Here's how the part is built. I have some questions about the finished solid (model axes, mm). Face numbers are marked on the shaded views. A direction names the side the tool comes from. Give positions to 0.01 mm unless a question says otherwise; leave off trailing zeros. Loops run counter-clockwise (first coordinate to the right, second up) from the corner with the lowest first, then second, coordinate; pieces in that order, holes last. Notation, with made-up numbers: (48.5, -30) - (106.5, -30) arc R19 ccw to (106.5, -2) - close; hole circle Ø6 at (30.5, 26.5). An arc over 180 degrees is marked (long way). Return JSON: item names as keys, results as strings. Group by question number.
(1) For P1, Ø2.5, axis at x = 6.35, z = 0, coming from the -Y side (3 decimals); P2, Ø1.5, axis at x = 11.5, y = 2.5, coming from the +Z side; P3, Ø5, axis at x = 27, y = 3, coming from the -Z side, each with a flat end and sliding along its axis, tell me the tip position at first contact or that it passes through.
(2) If we section it at C-C (x = 6.35): Please give me the cut outline in (y, z) (3 decimals).
(3) I need wall thicknesses on probe 1 along X at (y, z) = (2.85, 0); probe 2 along X at (y, z) = (-1.4, 0); probe 3 along X at (y, z) = (2.25, 0.5). Which ranges of each line are inside material? Lowest first, please. Write a range as [from, to].
(4) If we section it at B-B (y = 3.5): Please give me the cut outline in (x, z) (3 decimals).
(5) If we section it at A-A (z = 0): Please give me the cut outline in (x, y) (1 decimal), then the cut area to 3 significant figures.
(6) If we section it at D-D (x = 32.5): Please give me the cut outline in (y, z) (1 decimal).
(7) On a 3-axis mill with a long thin cutter (end or side, diameter ignored), from which of +Z, -Z, +X, -X, +Y, -Y can I reach the whole of each face in a straight line? I mean the marked faces 1 and 2. Say none if no direction works.
```python
from build123d import *

# Parameters (mm, degrees)
SKETCH1_R               = 4.7625
BOSS_EXTRUDE1_DEPTH     = 38.1
SKETCH2_R               = 2.0066
CUT_EXTRUDE1_DEPTH      = 7.9248
SKETCH3_R               = 1.1303
CUT_EXTRUDE2_DEPTH      = 8.6868
SKETCH4_R               = 5.084796601
SKETCH4_R_2             = 3.175
CUT_EXTRUDE3_DEPTH      = 9.525
SKETCH5_R               = 0.7874
CUT_EXTRUDE4_DEPTH      = 5.762500124
CUT_EXTRUDE4_DEPTH_BACK = 5.7625001


with BuildPart() as part:
    # Sketch1 → Boss-Extrude1 (new body)
    with BuildSketch(Plane(origin=(0, 0, 0), x_dir=(0, 0, -1), z_dir=(1, 0, 0))):
        Circle(SKETCH1_R)
    extrude(amount=BOSS_EXTRUDE1_DEPTH)

    # Sketch2 → Cut-Extrude1 (cut)
    with BuildSketch(Plane(origin=(38.1, 0, 0), x_dir=(0, 0, -1), z_dir=(1, 0, 0))):
        Circle(SKETCH2_R)
    extrude(amount=-CUT_EXTRUDE1_DEPTH, mode=Mode.SUBTRACT)

    # Sketch3 → Cut-Extrude2 (cut)
    with BuildSketch(Plane(origin=(0, 0, 0), x_dir=(1, 0, 0), z_dir=(0, 1, 0))):
        with Locations((34.1376, 0)):
            Circle(SKETCH3_R)
    extrude(amount=CUT_EXTRUDE2_DEPTH, mode=Mode.SUBTRACT)

    # Sketch4 → Cut-Extrude3 (cut)
    with BuildSketch(Plane.ZY):
        Circle(SKETCH4_R)
        Circle(SKETCH4_R_2, mode=Mode.SUBTRACT)
    extrude(amount=-CUT_EXTRUDE3_DEPTH, mode=Mode.SUBTRACT)

    # Sketch5 → Cut-Extrude4 (cut, two sides)
    with BuildSketch(Plane(origin=(0, 0, 0), x_dir=(1, 0, 0), z_dir=(0, 1, 0))) as cut_extrude4_sk:
        with Locations((6.35, 0)):
            Circle(SKETCH5_R)
    extrude(amount=CUT_EXTRUDE4_DEPTH, mode=Mode.SUBTRACT)
    extrude(cut_extrude4_sk.sketch, amount=-CUT_EXTRUDE4_DEPTH_BACK, mode=Mode.SUBTRACT)


solid = part.part
```
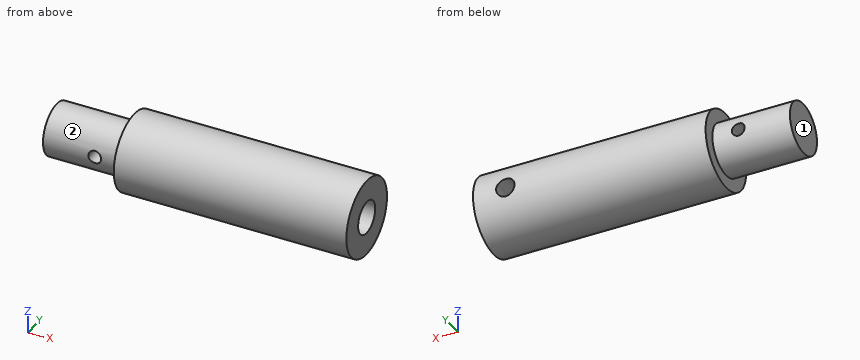
Values:
{
 "1": {"P1": "y = -3.175", "P2": "z = 4.43", "P3": "z = -4.74"},
 "2": {"outline": "(-3.076, -0.787) arc R3.175 ccw to (3.076, -0.787) - close; (-3.076, 0.787) - (3.076, 0.787) arc R3.175 ccw to start"},
 "3": {"probe 1": "[0, 5.56], [7.14, 33.01], [35.27, 38.1]", "probe 2": "[0, 5.56], [7.14, 30.18]", "probe 3": "[0, 5.74], [6.96, 33.12], [35.15, 38.1]"},
 "4": {"outline": "(9.525, -3.23) - (38.1, -3.23) - (38.1, 3.23) - (9.525, 3.23) - close; hole circle Ø2.261 at (34.138, 0)"},
 "5": {"outline": "(0, -3.2) - (5.6, -3.2) - (5.6, 3.2) - (0, 3.2) - close; (7.1, -3.2) - (9.5, -3.2) - (9.5, -4.8) - (38.1, -4.8) - (38.1, -2) - (30.2, -2) - (30.2, 2) - (33, 2) - (33, 4.8) - (9.5, 4.8) - (9.5, 3.2) - (7.1, 3.2) - close; (35.3, 2) - (38.1, 2) - (38.1, 4.8) - (35.3, 4.8) - close", "area": "285 mm2"},
 "6": {"outline": "circle Ø9.5 at (0, 0); hole circle Ø4 at (0, 0)"},
 "7": {"face 1": "+Z, -Z, -X, +Y, -Y", "face 2": "-X"}
}
